Geometry: see drawing. Coordinates: mm, zero at the bounding-box minimum. A direction names the side the tool comes from. Give positions to 0.01 mm unless a question says otherwise; leave off trailing zeros. Loops run counter-clockwise (first coordinate to the right, second up) from the corner with the lowest first, then second, coordinate; pieces in that order, holes last. Notation, with made-up numbers: M 89,13 L 128,13 A12 ccw 128,28 Z; hole C 3.25,-1.5 d7. An arc over 180 degrees is marked long. Answer in a Markdown table with one row per item.
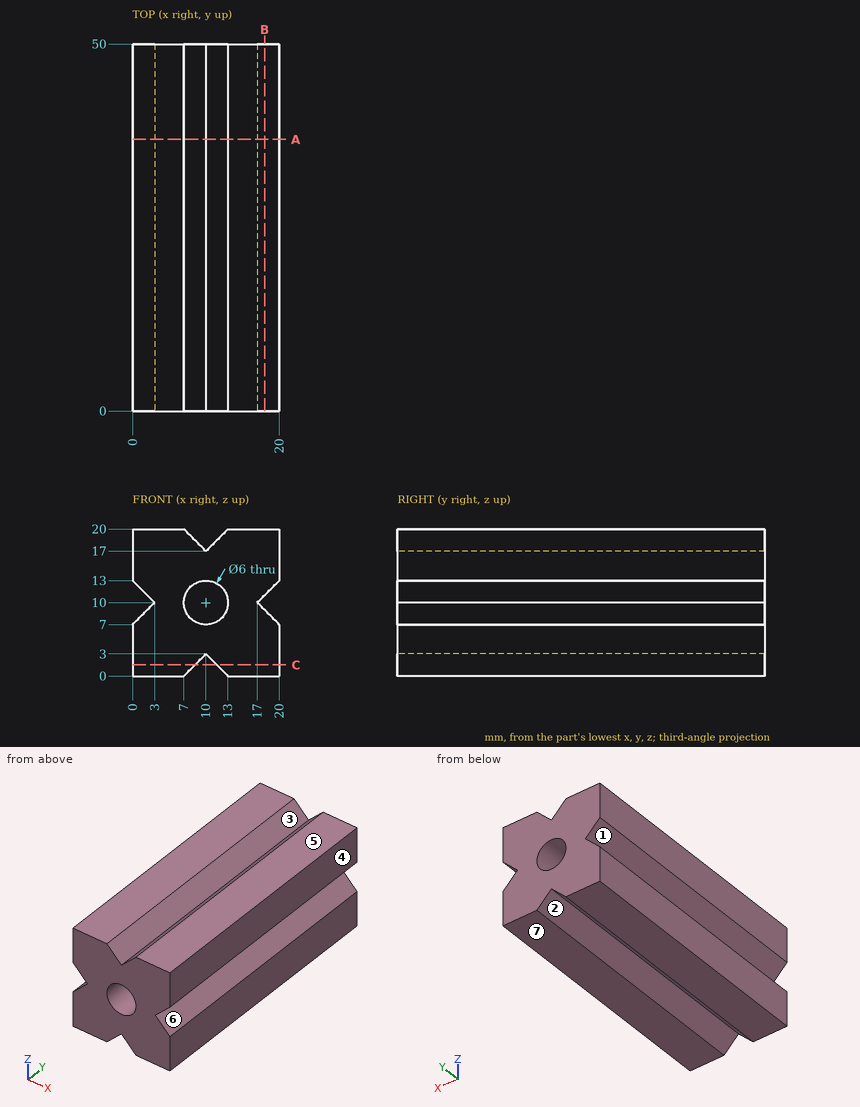
1) Section C-C, the plane z = 1.5. Return loops of the section in (x, y), then the cut area to 3 significant figures.
Reply:
| item | result |
|---|---|
| outline | M 0,0 L 8.5,0 L 8.5,50 L 0,50 Z; M 11.5,0 L 20,0 L 20,50 L 11.5,50 Z |
| area | 850 mm² |
2) Set-up query: the marked faces 1, 2 and 3. Return all of +Z, -Z, +X, -X, +Y, -Y with unobstructed straight access to the full face (end or side cutting, diameter ignored); none if empty.
Reply:
| item | result |
|---|---|
| face 1 | -X, +Y, -Y |
| face 2 | -Z, +Y, -Y |
| face 3 | +Z, +Y, -Y |
3) Material intervals for L1, parallel to X at y = 13, z = 2.25; L2, parallel to X at y = 24, z = 1; L3, parallel to Z at x = 8.5, y = 24.5, sorted ascending.
Reply:
| item | result |
|---|---|
| L1 | x = 0 to 9.25, 10.75 to 20 |
| L2 | x = 0 to 8, 12 to 20 |
| L3 | z = 1.5 to 7.4, 12.6 to 18.5 |
4) Section A-A, the plane y = 37. Return loops of the section in (x, z).
Reply:
| item | result |
|---|---|
| outline | M 0,0 L 7,0 L 10,3 L 13,0 L 20,0 L 20,7 L 17,10 L 20,13 L 20,20 L 13,20 L 10,17 L 7,20 L 0,20 L 0,13 L 3,10 L 0,7 Z; hole C 10,10 d6 |
5) Pull-direction query (Z, two-part tool) for the marked faces 4, 5, 6 and 7; classes: released by +Z, released by -Z, zero draft, split by the parting line, or undercut.
Reply:
| item | result |
|---|---|
| face 4 | zero draft |
| face 5 | released by +Z |
| face 6 | undercut |
| face 7 | released by -Z |
6) Section B-B, the plane x = 18. Return loops of the section in (y, z).
Reply:
| item | result |
|---|---|
| outline | M 0,0 L 50,0 L 50,9 L 0,9 Z; M 0,11 L 50,11 L 50,20 L 0,20 Z |
